from build123d import *

# Parameters (mm, degrees)
F0_R     = 20.6756
F0_R_2   = 5.9436
F1_DEPTH = 25.4
F0_R_3   = 3.0734
F2_DEPTH = 21.3868


with BuildPart() as f1:
    # F0 (on Front) → F1 (new body)
    with BuildSketch(Plane.XZ):
        with BuildLine():
            Line((271.580863, 23.272072), (167.052843, 23.272072))
            add(Edge.make_bspline(
                [(146.7104, 33.279704), (158.211127, 33.278), (155.84334, 23.444525), (167.052843, 23.272072)],
                knots=[0, 0, 0, 0, 22.670855, 22.670855, 22.670855, 22.670855], degree=3))
            add(Edge.make_bspline(
                [(146.7104, 33.279704), (135.209673, 33.278), (139.371195, 22.469644), (128.161692, 22.297191)],
                knots=[0, 0, 0, 0, 21.55621, 21.55621, 21.55621, 21.55621], degree=3))
            Line((128.161692, 22.297191), (23.633672, 22.297191))
            ThreePointArc((23.633672, 22.297191), (18.743023, 22.935671), (14.180203, 24.808314))
            ThreePointArc((14.180203, 24.808314), (-28.570281, -0.519307), (15.072395, -24.276605))
            ThreePointArc((15.072395, -24.276605), (16.798322, -23.325045), (18.613326, -22.556899))
            ThreePointArc((18.613326, -22.556899), (81.676421, -5.682276), (146.7104, 0))
            ThreePointArc((146.7104, 0), (211.744379, -5.682276), (274.807474, -22.556899))
            ThreePointArc((274.807474, -22.556899), (276.622478, -23.325045), (278.348405, -24.276605))
            ThreePointArc((278.348405, -24.276605), (321.973387, -1.131548), (280.316838, 25.393243))
            ThreePointArc((280.316838, 25.393243), (276.075766, 23.809958), (271.580863, 23.272072))
        make_face()
        Circle(F0_R, mode=Mode.SUBTRACT)
        with Locations((293.4208, 0)):
            Circle(F0_R, mode=Mode.SUBTRACT)
        with BuildLine():
            ThreePointArc((61.316134, 15.272072), (63.561198, 14.342136), (64.491134, 12.097072))
            Line((64.491134, 12.097072), (64.491134, 1.615122))
            ThreePointArc((64.491134, 1.615122), (63.797035, -0.36623), (62.018216, -1.48128))
            ThreePointArc((62.018216, -1.48128), (48.077329, -4.918229), (34.275062, -8.875302))
            ThreePointArc((34.275062, -8.875302), (31.242012, -8.220636), (30.215605, -5.292417))
            ThreePointArc((30.215605, -5.292417), (30.534281, 2.941109), (28.649913, 10.962433))
            ThreePointArc((28.649913, 10.962433), (28.999613, 13.896814), (31.615249, 15.272072))
            Line((31.615249, 15.272072), (61.316134, 15.272072))
        make_face(mode=Mode.SUBTRACT)
        with BuildLine():
            Line((83.525193, 15.272072), (123.526418, 15.272072))
            ThreePointArc((123.526418, 15.272072), (125.771482, 14.342136), (126.701418, 12.097072))
            Line((126.701418, 12.097072), (126.701418, 10.478448))
            ThreePointArc((126.701418, 10.478448), (125.837891, 8.301818), (123.717029, 7.309174))
            ThreePointArc((123.717029, 7.309174), (103.822564, 5.591163), (84.044681, 2.8386))
            ThreePointArc((84.044681, 2.8386), (81.471994, 3.549037), (80.350193, 5.970813))
            Line((80.350193, 5.970813), (80.350193, 12.097072))
            ThreePointArc((80.350193, 12.097072), (81.280129, 14.342136), (83.525193, 15.272072))
        make_face(mode=Mode.SUBTRACT)
        with Locations((146.7104, 23.1902)):
            Circle(F0_R_2, mode=Mode.SUBTRACT)
        with BuildLine():
            ThreePointArc((213.070607, 5.970813), (211.948806, 3.549037), (209.376119, 2.8386))
            ThreePointArc((209.376119, 2.8386), (189.598236, 5.591163), (169.703771, 7.309174))
            ThreePointArc((169.703771, 7.309174), (167.582909, 8.301818), (166.719382, 10.478448))
            Line((166.719382, 10.478448), (166.719382, 12.097072))
            ThreePointArc((166.719382, 12.097072), (167.649318, 14.342136), (169.894382, 15.272072))
            Line((169.894382, 15.272072), (209.895607, 15.272072))
            ThreePointArc((209.895607, 15.272072), (212.140671, 14.342136), (213.070607, 12.097072))
            Line((213.070607, 12.097072), (213.070607, 5.970813))
        make_face(mode=Mode.SUBTRACT)
        with BuildLine():
            ThreePointArc((261.805551, 15.272072), (264.421187, 13.896814), (264.770887, 10.962433))
            ThreePointArc((264.770887, 10.962433), (262.886519, 2.941109), (263.205195, -5.292417))
            ThreePointArc((263.205195, -5.292417), (262.178788, -8.220636), (259.145738, -8.875302))
            ThreePointArc((259.145738, -8.875302), (241.164238, -3.829591), (222.958148, 0.333559))
            ThreePointArc((222.958148, 0.333559), (221.131826, 1.435806), (220.415228, 3.445006))
            Line((220.415228, 3.445006), (220.415228, 12.097072))
            ThreePointArc((220.415228, 12.097072), (221.345164, 14.342136), (223.590228, 15.272072))
            Line((223.590228, 15.272072), (261.805551, 15.272072))
        make_face(mode=Mode.SUBTRACT)
    extrude(amount=F1_DEPTH)

    # F0 (on Front) → F2 (join)
    with BuildSketch(Plane.XZ):
        with Locations((146.7104, 23.1902)):
            Circle(F0_R_2)
        with Locations((146.7104, 23.1902)):
            Circle(F0_R_3, mode=Mode.SUBTRACT)
    extrude(amount=F2_DEPTH)


solid = f1.part
Design review of the part built by this model. Coordinates are the model's own, in mm. A direction names the side the tool comes from. Give positions to 0.01 mm unless a question says otherwise; leave off trailing zeros. Loops run counter-clockwise (first coordinate to the right, second up) from the corner with the lowest first, then second, coordinate; pieces in that order, holes last. Notation, with made-up numbers: M 22.25,5 L 42.25,5 A24 cw 42.25,15 Z; hole C 49.5,63 d3. An arc over 180 degrees is marked long. Answer as a JSON object with one key per item and string values.
Item 1: We need section A-A (x = 0). State the section outline as (y, z) points (3 decimals), and give its area (3 significant figures).
Output values:
{"outline": "M -25.4,-28.575 L 0,-28.575 L 0,-20.676 L -25.4,-20.676 Z; M -25.4,20.676 L 0,20.676 L 0,28.575 L -25.4,28.575 Z", "area": "401 mm2"}
Item 2: Wall thickness on line 1 along Z through (x, y) = (0, -10.25) (3 decimals); line 2 along Z through (x, y) = (39, -6.25); line 3 along X through (y, z) = (-11, -24): over which ranges is each line inside the solid? List them lowest first.
Output values:
{"line 1": "z = -28.575 to -20.676, 20.676 to 28.575", "line 2": "z = -15.8 to -7.46, 15.27 to 22.3", "line 3": "x = -15.51 to 15.53, 277.89 to 308.93"}
Item 3: We need section B-B (x = 178.5). State the section outline as (y, z) points.
Output values:
{"outline": "M -25.4,-1.35 L 0,-1.35 L 0,6.68 L -25.4,6.68 Z; M -25.4,15.27 L 0,15.27 L 0,23.27 L -25.4,23.27 Z"}
Item 4: We need section C-C (y = -13). Count the separate pieces of the cut face and the enclosed holes in it, and give its area (3 significant figures).
Output values:
{"separate pieces": "1", "enclosed holes": "7", "area": "7,330 mm2"}
Item 5: Machinability: for faces 1 (the face through (140.773, -23.365, 23.452)), 2 (the face through (146, -25.4, 5)), 3 (the face through (48.272, -12.522, -4.867)), 4 (the face through (276.137, -12.522, 23.825)), which of the approach directions +Z, -Z, +X, -X, +Y, -Y give a long, thin tool a straight path to every point of the face, cutting with its end or side? Answer none if there is none.
Output values:
{"face 1": "-Y", "face 2": "+Z, -Z, +X, -X, -Y", "face 3": "+Y, -Y", "face 4": "+Z, +Y, -Y"}
Item 6: For P1, Ø1.3, axis at y = -8.5, z = 11, coming from the -X side; P2, Ø1.5, axis at y = -9.5, z = -15.5, coming from the -X side; P3, Ø4.5, axis at y = -11.5, z = 7, coming from the +X side; P4, Ø3.5, axis at x = 146.71, z = 23.19, coming from the +Y side, all flat-tipped, find the tip position at first contact; note any pin that passes through.
Output values:
{"P1": "stops at x = -26.63", "P2": "stops at x = -24.47", "P3": "stops at x = 321.6", "P4": "passes through"}
